from build123d import *

# Parameters (mm, degrees)
F1_DEPTH = 19.05
F2_SIZE  = 12.7
F3_SIZE  = 12.7
F4_D     = 12.7
F6_DEPTH = 12.7
F8_D     = 19.05


with BuildPart() as f1:
    # F0 (on Right) → F1 (new body)
    with BuildSketch(Plane.YZ):
        Polygon((-31.75, 19.05), (-31.75, -19.05), (31.75, -19.05), (31.75, 19.05), (0, 19.05), align=None)
    extrude(amount=F1_DEPTH)

    # F2
    f2_edges = [f1.edges().sort_by_distance(p)[0] for p in [
        (9.525, -31.75, -19.05),
    ]]
    chamfer(f2_edges, length=F2_SIZE)

    # F3
    f3_edges = [f1.edges().sort_by_distance(p)[0] for p in [
        (9.525, 31.75, -19.05),
    ]]
    chamfer(f3_edges, length=F3_SIZE)

    # F4 (through all)
    with Locations(Plane(origin=(0, 0, 0), x_dir=(0, 1, 0), z_dir=(-1, 0, 0))):
        with Locations((-14.6544640884, 6.5692421049), (18.8520774245, 6.5692421049)):
            Hole(F4_D / 2)

    # F5 (on face) → F6 (join)
    with BuildSketch(Plane.XY.offset(19.05)):
        with BuildLine():
            Line((0, -31.75), (0, 0))
            Line((0, 0), (-31.75, 0))
            ThreePointArc((-31.75, 0), (-22.4506403027, -22.4506403027), (0, -31.75))
        make_face()
        with BuildLine():
            Line((-31.75, 0), (0, 0))
            Line((0, 0), (0, 31.75))
            ThreePointArc((0, 31.75), (-22.4506403027, 22.4506403027), (-31.75, 0))
        make_face()
    extrude(amount=-F6_DEPTH)

    # F8 (through all)
    with Locations(Plane(origin=(0, 0, 0), x_dir=(1, 0, 0), z_dir=(0, 0, -1))):
        with Locations((-15.875, 0)):
            Hole(F8_D / 2)


solid = f1.part
Read the model definition and answer for the solid it produces. Units are mm, in the model's axes. A direction names the side the tool comes from. Coordinates: 2 decimals unless noted, no trailing zeros. Write each loop counter-clockwise with the first axis right and the second up, starting at its lowest first coordinate (ties: lowest second). Pieces come first, ordered by that corner, then holes. Notation, with made-up numbers: (-21.5, 83) - (-9.5, 83) arc R20 ccw to (-9.5, 95) - close; hole circle Ø4 at (-34.5, 13.25). An arc over 180 degrees is marked (long way). One line per question, with ' | ' between items.
Q1. Determine the mould class of faces 3 (the flat face through (9, 0, -19.05)), 4 (the flat face through (9, -31.75, 7)), 5 (the cylindrical face through (9.658, 12.795, -8.477)) for opening direction Z: +Z half, -Z half, draft (parallel to the pull), parting line (faces both ways), or undercut.
Result set:
face 3: -Z half | face 4: draft | face 5: undercut
Q2. Find section B-B, the plane z = -4.5. Write down the section's boundary in (x, y).
Result set:
outline: (0, -31.75) - (19.05, -31.75) - (19.05, -20.66) - (0, -20.66) - close; (0, -8.65) - (19.05, -8.65) - (19.05, 12.85) - (0, 12.85) - close; (0, 24.86) - (19.05, 24.86) - (19.05, 31.75) - (0, 31.75) - close
Q3. Find section D-D, the plane z = 13. Write down the section's boundary in (x, y) (3 decimals).
Result set:
outline: (0, -31.75) - (19.05, -31.75) - (19.05, 31.75) - (0, 31.75) arc R31.75 ccw to start; hole circle Ø19.05 at (-15.875, 0)
Q4. Consider L1, parallel to Y at x = 8.5, z = -3; L2, parallel to Y at x = 11, z = -4.5; L3, parallel to X at y = -3, z = 9. Determine where each line is inside the solid, lowest interval first. Write a range as [from, to].
Result set:
L1: [-31.75, -19.91], [-9.4, 13.6], [24.1, 31.75] | L2: [-31.75, -20.66], [-8.65, 12.85], [24.86, 31.75] | L3: [-31.61, -24.92], [-6.83, 19.05]
Q5. Find section C-C, the plane y = -1.5. Write down the section's boundary in (x, z).
Result set:
outline: (-31.71, 6.35) - (-25.28, 6.35) - (-25.28, 19.05) - (-31.71, 19.05) - close; (-6.47, 6.35) - (0, 6.35) - (0, -19.05) - (19.05, -19.05) - (19.05, 19.05) - (-6.47, 19.05) - close
Q6. For faces 1 (the flat face through (-6, 0, 6.35)), 2 (the cylindrical face through (-24.96, -2.86, 12.79)), determine the directions among +Z, -Z, +X, -X, +Y, -Y from which every point of the face is accessible in a straight line to the end or side of a thin tool.
Result set:
face 1: -Z, -X, +Y, -Y | face 2: +Z, -Z
Q7. Each of these flat-tipped pins is pushed along its axis until it touches: P1, Ø1.5, axis at y = 11.5, z = -3, coming from the -X side; P2, Ø5, axis at x = -19, y = 12, coming from the -Z side; P3, Ø15, axis at x = -15.875, y = 0, coming from the -Z side; P4, Ø5, axis at y = -3.5, z = 9, coming from the -X side. Where does it stop, or does it pass through?
Result set:
P1: x = 0 | P2: z = 6.35 | P3: through | P4: x = -31.73
Q8. Find section A-A, the plane x = -14.5. Write down the section's boundary in (y, z), plus the area to 3 significant figures.
Result set:
outline: (-28.25, 6.35) - (-9.43, 6.35) - (-9.43, 19.05) - (-28.25, 19.05) - close; (9.43, 6.35) - (28.25, 6.35) - (28.25, 19.05) - (9.43, 19.05) - close | area: 478 mm^2
